from build123d import *

# Parameters (mm, degrees)
SKETCH1_R           = 3.175
BOSS_EXTRUDE1_DEPTH = 6.35
BOSS_EXTRUDE2_START = -6.35
BOSS_EXTRUDE2_DEPTH = 6.35
BOSS_EXTRUDE3_START = -6.35
SKETCH3_R           = 3.175
BOSS_EXTRUDE3_DEPTH = 6.35


with BuildPart() as part:
    # Sketch1 → Boss-Extrude1 (new body)
    with BuildSketch(Plane(origin=(0, 0, 0), x_dir=(1, 0, 0), z_dir=(0, 1, 0))):
        with BuildLine():
            Line((0, -6.35), (-76.2, -6.35))
            ThreePointArc((-76.2, -6.35), (-82.55, 0), (-76.2, 6.35))
            Line((-76.2, 6.35), (0, 6.35))
            ThreePointArc((0, 6.35), (6.35, 0), (0, -6.35))
        make_face()
        with Locations(Location((-76.2, 0, 0), (0, 0, 270))):
            Circle(SKETCH1_R, mode=Mode.SUBTRACT)
        with Locations(Location((0, 0, 0), (0, 0, 270))):
            Circle(SKETCH1_R, mode=Mode.SUBTRACT)
    extrude(amount=BOSS_EXTRUDE1_DEPTH)

    # Sketch2 → Boss-Extrude2 (add)
    with BuildSketch(Plane(origin=(0, 6.35, 0), x_dir=(1, 0, 0), z_dir=(0, 1, 0)).offset(BOSS_EXTRUDE2_START)):
        with BuildLine():
            Line((3.175, -5.499261314), (25.172045256, 7.200738686))
            ThreePointArc((25.172045256, 7.200738686), (27.340610585, 15.293934671), (19.247414599, 17.4625))
            Line((19.247414599, 17.4625), (0, 6.35))
            ThreePointArc((0, 6.35), (6.133628997, 1.643500936), (3.175, -5.499261314))
        make_face()
    extrude(amount=BOSS_EXTRUDE2_DEPTH)

    # Sketch3 → Boss-Extrude3 (add)
    with BuildSketch(Plane(origin=(0, 6.35, 0), x_dir=(1, 0, 0), z_dir=(0, 1, 0)).offset(BOSS_EXTRUDE3_START)):
        with BuildLine():
            Line((25.172045256, 17.4625), (47.169090512, 4.7625))
            ThreePointArc((47.169090512, 4.7625), (49.337655841, -3.330695986), (41.244459855, -5.499261314))
            Line((41.244459855, -5.499261314), (22.209729928, 5.490445134))
            Line((22.209729928, 5.490445134), (25.172045256, 7.200738686))
            ThreePointArc((25.172045256, 7.200738686), (28.134360585, 12.331619343), (25.172045256, 17.4625))
        make_face()
        with Locations(Location((44.206775184, -0.368380657, 0), (0, 0, 270))):
            Circle(SKETCH3_R, mode=Mode.SUBTRACT)
    extrude(amount=BOSS_EXTRUDE3_DEPTH)


solid = part.part
The model under review builds one solid part; all positions refer to its coordinate system, in mm. A direction names the side the tool comes from. Round coordinates to 2 decimals unless told otherwise and drop trailing zeros. Write each loop counter-clockwise with the first axis right and the second up, starting at its lowest first coordinate (ties: lowest second). Pieces come first, ordered by that corner, then holes. Notation, with made-up numbers: M -17.75,-22.5 L -8.75,-22.5 A21 ccw -8.75,-9.5 Z; hole C -9,-39 d9. An arc over 180 degrees is marked long. Use a Markdown table: item, result. Add a question column.
Q1. We need section C-C, the plane x = 39. State the section outline as (y, z) points, plus the area to 3 significant figures.
Q2. Insertion check: pin 1 (1 mm diameter, centred on y = 3, z = -7.5, fed in from +X); pin 2 (2 mm diameter, centred on y = 3.5, z = -15.5, fed in from +X); pin 3 (1 mm diameter, centred on x = 2, y = 2.5, fed in from -Z); pin 4 (5.5 mm diameter, centred on x = 44.21, z = 0.37, fed in from -Y). Each pin has a flat end and moves straight along its axis. Give the tip position at first contact, or say it passes through.
Q3. To check wall thickness, follow line 1 (X direction, y = 4.5, z = -0.5); line 2 (X direction, y = 3.5, z = -1.25); line 3 (Z direction, x = -30, y = 5.25). State the ranges of each line that lie inside material, in increasing order.
Q4. We need section A-A, the plane z = 0. State the section outline as (x, y) points (3 decimals), plus the area to 3 significant figures.
Q5. Machinability: for faces 1 (the face through (41.107, 3.131, -0.32)), 2 (the face through (31.86, 3.13, 0.08)), 3 (the face through (-39, 3, -6.35)), which of the approach directions +Z, -Z, +X, -X, +Y, -Y give a long, thin tool a straight path to every point of the face, cutting with its end or side? Answer none if there is none.
Q6. We need section B-B, the plane y = 1.5. Count the separate pieces of the cut face and the enclosed holes in it, plus the area to 3 significant figures.
Q7. The part is to be moulded in two halves that separate along Z. For faces 4 (the face through (-79.3, 3.13, -0.69)), 5 (the face through (-38, 3, 6.35)), 6 (the face through (-15, 0, -3)), say which applies: pulls with the +Z half, pulls with the -Z half, needs draft (parallel to the pull), parting line crosses it, or undercut.
Findings below:
| question | item | result |
|---|---|---|
| 1 | outline | M 0,-9.48 L 6.35,-9.48 L 6.35,4.2 L 0,4.2 Z |
| 1 | area | 86.9 mm² |
| 2 | pin 1 | stops at x = 43.29 |
| 2 | pin 2 | stops at x = 30.3 |
| 2 | pin 3 | stops at z = -7.79 |
| 2 | pin 4 | passes through |
| 3 | line 1 | x = -82.53 to -79.34, -73.06 to -3.14, 3.14 to 13.57, 30.85 to 41.15, 47.26 to 50.07 |
| 3 | line 2 | x = -82.43 to -79.12, -73.28 to -2.92, 2.92 to 14.87, 29.55 to 41.48, 46.94 to 49.91 |
| 3 | line 3 | z = -6.35 to 6.35 |
| 4 | outline | M -82.55,0 L -79.375,0 L -79.375,6.35 L -82.55,6.35 Z; M -73.025,0 L -3.175,0 L -3.175,6.35 L -73.025,6.35 Z; M 3.175,0 L 12.7,0 L 12.7,6.35 L 3.175,6.35 Z; M 31.719,0 L 41.053,0 L 41.053,6.35 L 31.719,6.35 Z; M 47.36,0 L 50.12,0 L 50.12,6.35 L 47.36,6.35 Z |
| 4 | area | 601 mm² |
| 5 | face 1 | +Y, -Y |
| 5 | face 2 | +Z, +Y, -Y |
| 5 | face 3 | -Z, -X, +Y, -Y |
| 6 | separate pieces | 1 |
| 6 | enclosed holes | 3 |
| 6 | area | 1,590 mm² |
| 7 | face 4 | undercut |
| 7 | face 5 | pulls with the +Z half |
| 7 | face 6 | needs draft |
